```python
from build123d import *

# Parameters (mm, degrees)
SKETCH1_W           = 34
SKETCH1_H           = 34.5
BOSS_EXTRUDE2_DEPTH = 13.5
SHELL1_T            = -3
SKETCH4_R           = 1.1
SKETCH4_R_2         = 2.5
CUT_EXTRUDE2_DEPTH  = 3
CHAMFER1_SIZE       = 0.6
SKETCH5_W           = 7.5
SKETCH5_H           = 7.5
CUT_EXTRUDE4_DEPTH  = 3
SKETCH6_W           = 34
SKETCH6_H           = 34.5
SKETCH6_W_2         = 31
SKETCH6_H_2         = 31.5
CUT_EXTRUDE5_DEPTH  = 4
FILLET1_R           = 0.8
CUT_EXTRUDE6_DEPTH  = 40.5
SKETCH8_W           = 34
SKETCH8_H           = 9.5
BOSS_EXTRUDE3_DEPTH = 8
LOFT1_START         = -17
LOFT1_DEPTH         = 34
SKETCH2_W           = 20
SKETCH2_H           = 4
CUT_EXTRUDE1_DEPTH  = 15


# Read off the part's stored shape, not the designer's step: Loft1
with BuildPart() as part:
    # Sketch1 → Boss-Extrude2 (new body)
    with BuildSketch(Plane.XY):
        Rectangle(SKETCH1_W, SKETCH1_H)
    extrude(amount=BOSS_EXTRUDE2_DEPTH)

    # Shell1
    shell1_openings = [part.faces().sort_by_distance(p)[0] for p in [
        (0, 0, 13.5),
    ]]
    offset(amount=SHELL1_T, openings=shell1_openings, kind=Kind.INTERSECTION)

    # Sketch4 → Cut-Extrude2 (cut)
    with BuildSketch(Plane.XY.offset(3)):
        with Locations((-10.5, 9.25)):
            Circle(SKETCH4_R)
        with Locations((10.5, 9.25)):
            Circle(SKETCH4_R)
        with Locations((10.5, -4.25)):
            Circle(SKETCH4_R)
        with Locations((-10.5, -4.25)):
            Circle(SKETCH4_R)
        with Locations((-9, 2.75)):
            Circle(SKETCH4_R_2)
        with Locations((9, 2.75)):
            Circle(SKETCH4_R_2)
    extrude(amount=-CUT_EXTRUDE2_DEPTH, mode=Mode.SUBTRACT)

    # Chamfer1
    chamfer1_edges = [part.edges().sort_by_distance(p)[0] for p in [
        (-11.5, 2.75, 3),
        (6.5, 2.75, 3),
    ]]
    chamfer(chamfer1_edges, length=CHAMFER1_SIZE)

    # Sketch5 → Cut-Extrude4 (cut)
    with BuildSketch(Plane.XY.offset(3)):
        with Locations((0, 2.75)):
            Rectangle(SKETCH5_W, SKETCH5_H)
    extrude(amount=-CUT_EXTRUDE4_DEPTH, mode=Mode.SUBTRACT)

    # Sketch6 → Cut-Extrude5 (cut)
    with BuildSketch(Plane.XY.offset(13.5)):
        Rectangle(SKETCH6_W, SKETCH6_H)
        Rectangle(SKETCH6_W_2, SKETCH6_H_2, mode=Mode.SUBTRACT)
    extrude(amount=-CUT_EXTRUDE5_DEPTH, mode=Mode.SUBTRACT)

    # Fillet1
    fillet1_edges = [part.edges().sort_by_distance(p)[0] for p in [
        (15.5, -15.75, 11.5),
        (-15.5, -15.75, 11.5),
        (-15.5, 15.75, 11.5),
        (15.5, 15.75, 11.5),
    ]]
    fillet(fillet1_edges, radius=FILLET1_R)

    # Sketch7 → Cut-Extrude6 (cut, through all)
    with BuildSketch(Plane.XZ.offset(15.75)):
        Polygon((-15.5, 10), (-15.2, 10.3), (-15.2, 10.7), (-15.5, 11), align=None)
        Polygon((15.5, 10), (15.2, 10.3), (15.2, 10.7), (15.5, 11), align=None)
    extrude(amount=-CUT_EXTRUDE6_DEPTH, mode=Mode.SUBTRACT)

    # Sketch8 → Boss-Extrude3 (add)
    with BuildSketch(Plane.XZ.offset(17.25)):
        with Locations((0, 4.75)):
            Rectangle(SKETCH8_W, SKETCH8_H)
    extrude(amount=BOSS_EXTRUDE3_DEPTH)

    # Loft1 outline → Loft1 (add)
    with BuildSketch(Plane.YZ.offset(LOFT1_START)):
        with BuildLine():
            add(Edge.make_bspline(
                [(-27.448962768, 19.266529653), (-23.634638761, 16.661774183), (-19.340130821, 13.729106946), (-17.622252945, 9.933560294), (-17.457544345, 9.499999999)],
                knots=[0, 0, 0, 0, 0.544121998, 0.612621328, 0.612621328, 0.612621328, 0.612621328], degree=3))
            Line((-27.448962768, 19.266529653), (-29.418578274, 18.919233298))
            add(Edge.make_bspline(
                [(-29.418578274, 18.919233298), (-28.949482113, 15.724623902), (-28.092684774, 9.889716149), (-26.137682382, 3.173259559), (-25.25, 0.131617347)],
                knots=[0, 0, 0, 0, 0.544121998, 0.993830941, 0.993830941, 0.993830941, 0.993830941], degree=3))
            Line((-25.25, 0.131617347), (-25.25, 9.5))
            Line((-25.25, 9.5), (-17.457544345, 9.499999999))
        make_face()
    extrude(amount=LOFT1_DEPTH)

    # Sketch2 → Cut-Extrude1 (cut)
    with BuildSketch(Plane(origin=(0, -14.25, 0), x_dir=(1, 0, 0), z_dir=(0, 1, 0))):
        with Locations((0, -5)):
            Rectangle(SKETCH2_W, SKETCH2_H)
    extrude(amount=-CUT_EXTRUDE1_DEPTH, mode=Mode.SUBTRACT)


solid = part.part
```
For this review, take the finished solid that the model builds, in its own axes (mm). A direction names the side the tool comes from. Round coordinates to 2 decimals unless told otherwise and drop trailing zeros. Write each loop counter-clockwise with the first axis right and the second up, starting at its lowest first coordinate (ties: lowest second). Pieces come first, ordered by that corner, then holes.
1) Take a section at A-A on y = -4.25. Give the boundary of the cut face in (x, z).
Answer below:
outline: (-17, 0) - (-11.6, 0) - (-11.6, 3) - (-14, 3) - (-14, 13.5) - (-15.5, 13.5) - (-15.5, 11) - (-15.2, 10.7) - (-15.2, 10.3) - (-15.5, 10) - (-15.5, 9.5) - (-17, 9.5) - close; (-9.4, 0) - (9.4, 0) - (9.4, 3) - (-9.4, 3) - close; (11.6, 0) - (17, 0) - (17, 9.5) - (15.5, 9.5) - (15.5, 10) - (15.2, 10.3) - (15.2, 10.7) - (15.5, 11) - (15.5, 13.5) - (14, 13.5) - (14, 3) - (11.6, 3) - close
2) For line 1 along X through (y, z) = (-2.5, 6); line 2 along Y through (x, z) = (-2.5, 12.25); line 3 along Y through (x, z) = (10.5, 1.45), list the stretches that pass through material, from the lowest coordinate up.
Answer below:
line 1: x = -17 to -14, 14 to 17
line 2: y = -28.35 to -19, -15.75 to -14.25, 14.25 to 15.75
line 3: y = -25.63 to -5.35, -3.15 to 0.75, 4.75 to 8.15, 10.35 to 17.25
3) Take a section at C-C on y = -12. Give the boundary of the cut face in (x, z).
Answer below:
outline: (-17, 0) - (17, 0) - (17, 9.5) - (15.5, 9.5) - (15.5, 10) - (15.2, 10.3) - (15.2, 10.7) - (15.5, 11) - (15.5, 13.5) - (14, 13.5) - (14, 3) - (-14, 3) - (-14, 13.5) - (-15.5, 13.5) - (-15.5, 11) - (-15.2, 10.7) - (-15.2, 10.3) - (-15.5, 10) - (-15.5, 9.5) - (-17, 9.5) - close
4) Take a section at B-B on y = 2.75. State how many separate pieces and enclosed holes the cut face has, then the cut area to 3 significant figures.
Answer below:
separate pieces: 4
enclosed holes: 0
area: 99.4 mm2
5) Machinability: for faces 4 (the face through (-14, 0, 8)), 5 (the face through (0, 15.75, 12)), 6 (the face through (0, -21, 7)), 7 (the face through (0, 17.25, 5)), 8 (the face through (0, -1, 2)), which of the approach directions +Z, -Z, +X, -X, +Y, -Y give a long, thin tool a straight path to every point of the face, cutting with its end or side? Answer none if there is none.
Answer below:
face 4: +Z
face 5: +Z, +X, -X, +Y
face 6: -Y
face 7: +Z, -Z, +X, -X, +Y
face 8: +Z, -Z
6) Insertion check: pin 1 Ø8.5 at (x, y) = (-2, -15) entering from +Z; pin 2 Ø1.2 at (y, z) = (-4.5, 13) entering from +X; pin 3 Ø2 at (x, z) = (5, 11) entering from +Y. Each pin has a flat end and moves straight along its axis. Give the tip position at first contact, or say it passes through.
Answer below:
pin 1: stops at z = 13.5
pin 2: stops at x = 15.5
pin 3: stops at y = 15.75
7) Mouldability with a two-part tool opening along Z and no side actions: class faces 1 (the face through (3.75, 3, 2)), 2 (the face through (0, -4, 0)), 3 (the face through (0, -6, 3)) as +Z half, -Z half, draft (parallel to the pull), parting line (faces both ways), or undercut.
Answer below:
face 1: draft
face 2: -Z half
face 3: undercut
